Autodesk Inventor part; units mm, degrees
ref_plane "Work Plane1" through (-9.8694, 0, 0) normal (0, -0.866, -0.5) x (1, 0, 0)
ref_plane "YZ Plane" through (0, 0, 0) normal (1, 0, 0) x (0, 1, 0)
ref_plane "XZ Plane" through (0, 0, 0) normal (0, 1, 0) x (-1, 0, 0)
sketch "Sketch1" plane through (0, 0, 0) normal (1, 0, 0) x (0, 1, 0)
  line L0 (-4.5754, 0) -> (-2.2877, 3.9624)
  line L1 (-2.2877, 3.9624) -> (2.2877, 3.9624)
  line L2 (2.2877, 3.9624) -> (4.5754, 0)
  line L3 (4.5754, 0) -> (2.2877, -3.9624)
  line L4 (2.2877, -3.9624) -> (-2.2877, -3.9624)
  line L5 (-2.2877, -3.9624) -> (-4.5754, 0)
  point P0 (0, 0)
  point P1 (0, 0)
  dimension "d0" = 9.1508
extrude "Body" add sketch "Sketch1" along normal blind 2.4892
sketch "Sketch2" plane through (0, 0, 0) normal (0, 0, 1) x (1, 0, 0)
  line L0 (0, 2.2877) -> (0, 4.5754)
  line L1 (0, 4.5754) -> (2.4892, 4.5754)
  line L2 (2.4892, 2.2877) -> (2.4892, 4.5754)
  line L3 (-0.4978, 0) -> (2.987, 0)
  line L4 (0.3539, 4.5754) -> (0, 3.9624)
  line L5 (2.1353, 4.5754) -> (2.4892, 3.9624)
  dimension "d3" = 30
  dimension "d4" = 30
  dimension "d5" = 7.9248
  dimension "d6" = 7.9248
revolve "Chamfer1" cut sketch "Sketch2" angle 360 about axis through (-10, 0, 0) along (1, 0, 0)
sketch "Sketch3" plane through (2.4892, 0, 0) normal (1, 0, 0) x (0, 0, -1)
  arc A0 (-1.9812, -3.4315) -> (1.9812, -3.4315) centre (0, 0) ccw
hole "Thread" at (2.4892, 0, 0) direction (-1, 0, 0) diameter 2.5502 end through all
chamfer "Chamfer2" distance 0.3125 angle 30 1 edges at (2.4892, 0, 1.2751) measured on face at (2.4892, 3.0491, -0.0512)
chamfer "Chamfer3" distance 0.3125 angle 30 1 edges at (0, 0, 1.2751) measured on face at (0, -3.0491, -0.0512)
ref_plane "Work Plane1" through (-9.8694, 0, 0) normal (0, -0.866, -0.5) x (1, 0, 0)
equation "\"d0\" = 1.1547 * SW"
equation "\"d1\" = KOH"
equation "\"d3\" = ANG1"
equation "\"d4\" = ANG2"
equation "\"d5\" = SW0"
equation "\"d6\" = SW01"
equation "\"d8\" = -0.5 * GD1 + 0.5 * NND"
equation "\"d40\" = -0.5 * GD1 + 0.5 * NND"
equation "\"d10\" = -0.5 * GD1 + 0.5 * NND"
equation "\"d41\" = -0.5 * GD1 + 0.5 * NND"
equation "\"ANG1\" = 30deg"
equation "\"ANG2\" = 30deg"
equation "\"NND\" = 3.175"
equation "\"KOH\" = 2.4892"
equation "\"SW\" = 7.9248"
equation "\"SW0\" = SW"
equation "\"SW01\" = SW"
equation "\"THREADDIA\" = 3.175"
equation "\"TOA\" = 30deg"
equation "\"E0\" = 1.155 * SW"
properties part number "ANSI B18.6.3 - 5 - 44" material "Steel, Mild"
Input: part model. Units: mm. Frame: model coordinates. Give positions to 0.01 mm unless a question says otherwise; leave off trailing zeros. Write each loop counter-clockwise with the first axis right and the second up, starting at its lowest first coordinate (ties: lowest second). Pieces come first, ordered by that corner, then holes. Notation, with made-up numbers: M 38,15.5 L 61,15.5 A12 cw 61,26.5 Z; hole C 14.25,1.5 d5. An arc over 180 degrees is marked long. Use one line per item in the form item = value.
1. Mould query, pull axis Z, two halves, no side actions, for faces 1 (the face through (2.403, -4.111, -0.01)), 2 (the face through (1.227, -3.416, -2.009)), 3 (the face through (1.23, -0.383, -1.216)). Classes: released by +Z, released by -Z, zero draft, split by the parting line, or undercut.
Outcome:
face_1 = split by the parting line
face_2 = released by -Z
face_3 = undercut
2. First-contact query: P1, Ø3, axis at y = 0, z = 0, coming from the -X side; P2, Ø1, axis at y = 0, z = -0.5, coming from the -X side. Flat tips, straight axial feed; report the tip coordinate or a pass-through.
Outcome:
P1 = 0.05
P2 = through
3. Cut plane A-A on x = 1.05. Return loops of the section in (y, z).
Outcome:
outline = M -4.58,0 L -2.29,-3.96 L 2.29,-3.96 L 4.58,0 L 2.29,3.96 L -2.29,3.96 Z; hole C 0,0 d2.55
4. Ray query, L1, parallel to Z at x = 1.8, y = 0; L2, parallel to Z at x = 1.2, y = -0.5; L3, parallel to Y at x = 1.85, z = 0.5. Return the intervals inside material, ascending.
Outcome:
L1 = -3.96 to -1.28, 1.28 to 3.96
L2 = -3.96 to -1.17, 1.17 to 3.96
L3 = -4.29 to -1.17, 1.17 to 4.29
